Here's how the part is built. I have some questions about the finished solid (model axes, mm). A direction names the side the tool comes from. Give positions to 0.01 mm unless a question says otherwise; leave off trailing zeros. Write each loop counter-clockwise with the first axis right and the second up, starting at its lowest first coordinate (ties: lowest second). Pieces come first, ordered by that corner, then holes. Notation, with made-up numbers: (-12.75, -1.5) - (15.25, -1.5) arc R35 cw to (15.25, 35.5) - close; hole circle Ø7 at (23, -27.5). An arc over 180 degrees is marked (long way). Use a Markdown table: item, result.
```python
from build123d import *

# Parameters (mm, degrees)
F0_W     = 248.539
F0_H     = 38.227
F1_DEPTH = 38.227
F2_R     = 8.763
F2_R_2   = 3.937
F3_DEPTH = 19.05
F5_DEPTH = 38.228


with BuildPart() as f1:
    # F0 (on Top) → F1 (new body)
    with BuildSketch(Plane.XY):
        Rectangle(F0_W, F0_H)
    extrude(amount=F1_DEPTH)

    # F2 (on face) → F3 (cut)
    with BuildSketch(Plane.XY.offset(38.227)):
        with Locations((-107.6706, 0)):
            Circle(F2_R)
        Circle(F2_R_2)
        with Locations((107.6706, 0)):
            Circle(F2_R)
    extrude(amount=-F3_DEPTH, mode=Mode.SUBTRACT)

    # F4 (on face) → F5 (cut, through all)
    with BuildSketch(Plane.XY.offset(38.227)):
        with BuildLine():
            Line((-37.973, 4.572), (-63.3476, 4.572))
            ThreePointArc((-63.3476, 4.572), (-67.9196, 0), (-63.3476, -4.572))
            Line((-63.3476, -4.572), (-37.973, -4.572))
            ThreePointArc((-37.973, -4.572), (-33.401, 0), (-37.973, 4.572))
        make_face()
        with BuildLine():
            ThreePointArc((37.973, 4.572), (33.401, 0), (37.973, -4.572))
            Line((37.973, -4.572), (63.3476, -4.572))
            ThreePointArc((63.3476, -4.572), (67.9196, 0), (63.3476, 4.572))
            Line((63.3476, 4.572), (37.973, 4.572))
        make_face()
    extrude(amount=-F5_DEPTH, mode=Mode.SUBTRACT)


solid = f1.part
```
Item 1: If we section it at B-B, the plane y = 0: Write out the boundary of the cut face in (x, z), plus the area to 3 significant figures.
Values:
| item | result |
|---|---|
| outline | (-124.27, 0) - (-67.92, 0) - (-67.92, 38.23) - (-98.91, 38.23) - (-98.91, 19.18) - (-116.43, 19.18) - (-116.43, 38.23) - (-124.27, 38.23) - close; (-33.4, 0) - (33.4, 0) - (33.4, 38.23) - (3.94, 38.23) - (3.94, 19.18) - (-3.94, 19.18) - (-3.94, 38.23) - (-33.4, 38.23) - close; (67.92, 0) - (124.27, 0) - (124.27, 38.23) - (116.43, 38.23) - (116.43, 19.18) - (98.91, 19.18) - (98.91, 38.23) - (67.92, 38.23) - close |
| area | 6,040 mm2 |
Item 2: Will these pins go through, and if not, where does the flat tip stop? pin 1 Ø4 at (x, y) = (-50, -12) entering from -Z; pin 2 Ø16 at (x, y) = (107.67, 0) entering from +Z.
Values:
| item | result |
|---|---|
| pin 1 | stops at z = 0 |
| pin 2 | stops at z = 19.18 |
Item 3: I need wall thicknesses on line 1 along Y through (x, z) = (0, 29); line 2 along X through (y, z) = (-6, 32); line 3 along X through (y, z) = (-8, 20). Which ranges of each line are inside material? Lowest first, please. Write a range as [from, to].
Values:
| item | result |
|---|---|
| line 1 | y = [-19.11, -3.94], [3.94, 19.11] |
| line 2 | x = [-124.27, -114.06], [-101.28, 101.28], [114.06, 124.27] |
| line 3 | x = [-124.27, -111.25], [-104.09, 104.09], [111.25, 124.27] |
Item 4: If we section it at D-D, the plane z = 16: Write out the boundary of the cut face in (x, y), plus the area to 3 significant figures.
Values:
| item | result |
|---|---|
| outline | (-124.27, -19.11) - (124.27, -19.11) - (124.27, 19.11) - (-124.27, 19.11) - close; hole (-63.35, -4.57) - (-37.97, -4.57) arc R4.57 ccw to (-37.97, 4.57) - (-63.35, 4.57) arc R4.57 ccw to start; hole (37.97, -4.57) - (63.35, -4.57) arc R4.57 ccw to (63.35, 4.57) - (37.97, 4.57) arc R4.57 ccw to start |
| area | 8,910 mm2 |
Item 5: If we section it at C-C, the plane x = 0: Write out the boundary of the cut face in (y, z).
Values:
| item | result |
|---|---|
| outline | (-19.11, 0) - (19.11, 0) - (19.11, 38.23) - (3.94, 38.23) - (3.94, 19.18) - (-3.94, 19.18) - (-3.94, 38.23) - (-19.11, 38.23) - close |
Item 6: Thinking about a two-plate mould opening in X: for faces 4 (the flat face through (50, -4.572, 19)), 5 (the flat face through (124.27, 0, 19)), 6 (the flat face through (-2, -19.114, 19)), which applies, +X half, -X half, draft (parallel to the pull), parting line (faces both ways), or undercut?
Values:
| item | result |
|---|---|
| face 4 | undercut |
| face 5 | +X half |
| face 6 | draft |
Item 7: For faces 1 (the cylindrical face through (67.92, -0.1, 19.38)), 2 (the cylindrical face through (-99.31, 2.63, 28.84)), 3 (the flat face through (-2, 5, 38.227)), which set-ups out of +Z, -Z, +X, -X, +Y, -Y let a thin tool reach every point of the face, with its end or its side?
Values:
| item | result |
|---|---|
| face 1 | +Z, -Z |
| face 2 | +Z |
| face 3 | +Z, +X, -X, +Y, -Y |
Item 8: If we section it at A-A, the plane z = 25.5: Write out the boundary of the cut face in (x, y).
Values:
| item | result |
|---|---|
| outline | (-124.27, -19.11) - (124.27, -19.11) - (124.27, 19.11) - (-124.27, 19.11) - close; hole circle Ø17.53 at (-107.67, 0); hole (-63.35, -4.57) - (-37.97, -4.57) arc R4.57 ccw to (-37.97, 4.57) - (-63.35, 4.57) arc R4.57 ccw to start; hole circle Ø7.87 at (0, 0); hole (37.97, -4.57) - (63.35, -4.57) arc R4.57 ccw to (63.35, 4.57) - (37.97, 4.57) arc R4.57 ccw to start; hole circle Ø17.53 at (107.67, 0) |
